```python
from build123d import *

# Parameters (mm, degrees)
F0_R     = 279.4
F1_DEPTH = 25.4
F2_R     = 13.3406236018
F6_R     = 76.3831689613
F7_DEPTH = 25.4


# Not quite as in the source:
# - a fillet or chamfer that OpenCascade refuses, or shapes differently, is made with other operations: its cross-section is extruded or revolved along the edge and cut away or added


with BuildPart() as f1:
    # F0 (on Front) → F1 (new body)
    with BuildSketch(Plane.XZ):
        Circle(F0_R)
    extrude(amount=F1_DEPTH)

    # F2 (on Top) → F3 (revolve, cut)
    with BuildSketch(Plane.XY):
        with Locations((278.8262367249, -11.0273361206)):
            Circle(F2_R)
    revolve(axis=Axis((0, 0, 0), (0, 1, 0)), mode=Mode.SUBTRACT)

    # F4: chamfer of 5.08 on 1 edges, made by hand

    # F4_s1 → F4_t2 (revolve, cut)
    with BuildSketch(Plane.XY):
        Polygon((279.4, -20.32), (274.32, -25.4), (279.4, -25.4), align=None)
    revolve(axis=Axis((0, -25.4, 0), (0, -1, 0)), mode=Mode.SUBTRACT)

    # F6 (on face) → F7 (cut)
    with BuildSketch(Plane(origin=(0, 0, 0), x_dir=(-1, 0, 0), z_dir=(0, 1, 0))):
        with Locations((-138.2894814014, -41.8609678745)):
            Circle(F6_R)
        with Locations((32.8920790944, 140.6926879071)):
            Circle(F6_R)
        with Locations((105.3974023071, -98.8317200326)):
            Circle(F6_R)
    extrude(amount=-F7_DEPTH, mode=Mode.SUBTRACT)


solid = f1.part
```
Here's how the part is built. I have some questions about the finished solid (model axes, mm). Give positions to 0.01 mm unless a question says otherwise; leave off trailing zeros. Loops run counter-clockwise (first coordinate to the right, second up) from the corner with the lowest first, then second, coordinate; pieces in that order, holes last. Notation, with made-up numbers: M -35,21.25 L 3,21.25 A22 ccw 3,51.25 Z; hole C 59.5,12.5 d9. An arc over 180 degrees is marked long. Return JSON: item names as keys, results as strings.
Item 1: Imagine slicing it at C-C on y = -6.5. List the corners of the cut face in (x, z) for me, then the cut area to 3 significant figures.
A:
{"outline": "C 0,0 d532.55; hole C -105.4,-98.83 d152.77; hole C -32.89,140.69 d152.77; hole C 138.29,-41.86 d152.77", "area": "168,000 mm^2"}
Item 2: I'm going to push flat-ended pins straight in: pin 1 Ø10 at (x, y) = (-177.5, -6) entering from -Z; pin 2 Ø8 at (x, y) = (153.5, -16.5) entering from +Z; pin 3 Ø1 at (y, z) = (-13.5, 179.5) entering from -X. Where does each tip first touch, or does it pass through?
A:
{"pin 1": "stops at z = -204.73", "pin 2": "stops at z = 222.19", "pin 3": "stops at x = -196.4"}
Item 3: Thinking about a two-plate mould opening in Z: for faces 1 (the cylindrical face through (-22.949, -12.522, 216.426)), 2 (the flat face through (-4, 0, 4)), which applies, released by +Z, released by -Z, zero draft, split by the parting line, or undercut?
A:
{"face 1": "undercut", "face 2": "zero draft"}
Item 4: Imagine slicing it at A-A on z = 0. List the corners of the cut face in (x, y) for me, then the cut area to 3 significant figures.
A:
{"outline": "M -275.72,-24 L -274.32,-25.4 L 74.4,-25.4 L 74.4,0 L -271.32,0 A13.34 cw Z; M 202.18,-25.4 L 274.32,-25.4 L 275.72,-24 A13.34 cw 271.32,0 L 202.18,0 Z", "area": "10,400 mm^2"}
Item 5: Imagine slicing it at B-B on x = 0. List the corners of the cut face in (y, z) for me, then the cut area to 3 significant figures.
A:
{"outline": "M -25.4,-274.32 L -24,-275.72 A13.34 cw 0,-271.32 L 0,71.75 L -25.4,71.75 Z; M -25.4,209.63 L 0,209.63 L 0,271.32 A13.34 cw -24,275.72 L -25.4,274.32 Z", "area": "10,100 mm^2"}
Item 6: Imagine slicing it at D-D on x = -77. State how many separate pieces and enclosed holes the cut face has, then the cut area to 3 significant figures.
A:
{"separate pieces": "3", "enclosed holes": "0", "area": "6,280 mm^2"}
Item 7: Please list where these lines run through material, in increasing order: line 1 (X direction, y = -12.75, z = -89); line 2 (Z direction, x = -90, y = -5); line 3 (X direction, y = -14.5, z = -75.5).
A:
{"line 1": "x = -250.24 to -181.15, -29.65 to 78.19, 198.39 to 250.24", "line 2": "z = -251.29 to -173.65, -24.02 to 89.97, 191.42 to 251.29", "line 3": "x = -255 to -178.13, -32.66 to 69.71, 206.87 to 255"}
